from build123d import *

# Parameters (mm, degrees)
SKETCH1_R           = 11
BOSS_EXTRUDE2_DEPTH = 7


with BuildPart() as part:
    # Sketch1 → Boss-Extrude2 (new body)
    with BuildSketch(Plane.XY):
        with BuildLine():
            ThreePointArc((20.169463689, 41.588983826), (18.10306117, 49.087649082), (10.604395914, 47.021246564))
            Line((10.604395914, 47.021246564), (-12.118876528, 7.010361333))
            ThreePointArc((-12.118876528, 7.010361333), (-19.668266357, -0.440838827), (-29.907048562, -3.212302261))
            Line((-29.907048562, -3.212302261), (-46.101848355, -3.327223978))
            ThreePointArc((-46.101848355, -3.327223978), (-51.562681703, -8.866113681), (-46.023791999, -14.326947029))
            Line((-46.023791999, -14.326947029), (-0.01171274, -14.000435605))
            ThreePointArc((-0.01171274, -14.000435605), (10.215910802, -16.8127989), (17.735459644, -24.294112676))
            Line((17.735459644, -24.294112676), (25.932384666, -38.261759848))
            ThreePointArc((25.932384666, -38.261759848), (33.459620532, -40.221535401), (35.419396085, -32.694299535))
            Line((35.419396085, -32.694299535), (12.130589268, 6.990074273))
            ThreePointArc((12.130589268, 6.990074273), (9.452355555, 17.253637727), (12.171588918, 27.506414937))
            Line((12.171588918, 27.506414937), (20.169463689, 41.588983826))
        make_face()
        with BuildLine():
            Line((6.354309168, 34.829758236), (12.626103421, 45.873063758))
            ThreePointArc((12.626103421, 45.873063758), (16.954878364, 47.065941576), (18.147756182, 42.737166632))
            Line((18.147756182, 42.737166632), (11.875961929, 31.69386111))
            ThreePointArc((11.875961929, 31.69386111), (7.547186985, 30.500983292), (6.354309168, 34.829758236))
        make_face(mode=Mode.SUBTRACT)
        with BuildLine():
            ThreePointArc((-46.040290274, -12.002005566), (-49.23774024, -8.849615406), (-46.08535008, -5.652165441))
            Line((-46.08535008, -5.652165441), (-33.38566983, -5.56204583))
            ThreePointArc((-33.38566983, -5.56204583), (-30.188219864, -8.71443599), (-33.340610024, -11.911885955))
            Line((-33.340610024, -11.911885955), (-46.040290274, -12.002005566))
        make_face(mode=Mode.SUBTRACT)
        Circle(SKETCH1_R, mode=Mode.SUBTRACT)
        with BuildLine():
            ThreePointArc((33.414186854, -33.871058192), (32.282861875, -38.216326169), (27.937593898, -37.085001191))
            Line((27.937593898, -37.085001191), (21.509707901, -26.13181528))
            ThreePointArc((21.509707901, -26.13181528), (22.641032879, -21.786547303), (26.986300856, -22.917872281))
            Line((26.986300856, -22.917872281), (33.414186854, -33.871058192))
        make_face(mode=Mode.SUBTRACT)
    extrude(amount=BOSS_EXTRUDE2_DEPTH)


solid = part.part
Build history of the part. All positions in model axes, mm. A direction names the side the tool comes from. Round coordinates to 2 decimals unless told otherwise and drop trailing zeros. Order: outer loops, then holes, each group sorted by start corner. A loop starts at its lowest first (then second) coordinate and runs counter-clockwise, first axis right, second up. Notation, with made-up numbers: M 12.25,51.5 L 34.25,51.5 A29 cw 34.25,80.5 Z; hole C -37.5,-5 d1. An arc over 180 degrees is marked long. Use CSV: the item, a comma, the result in double quotes. Start each with the question number.
(1) Drill centre lines: probe 1 along Y at (x, z) = (-45, 1.5); probe 2 along Y at (x, z) = (0, 2.5); probe 3 along Y at (x, z) = (6.5, 3). Where is each one in solid material? Low to high.
(2) Mould opens along Y. For faces 4 (the face through (21.777, -31.18, 3.451)), 5 (the face through (-19.538, -0.366, 3.451)), 6 (the face through (9.446, 40.274, 3.451)), 7 (the face through (-51.562, -8.745, 3.451)) say: +Y half, -Y half, draft (parallel to the pull), parting line (faces both ways), or undercut.
(3) Tool access for faces 1 (the face through (-0.598, 27.296, 3.451)), 2 (the face through (23.94, -13.13, 3.45)), 3 (the face through (24.77, -31.69, 3.45)): list every direction of +Z, -Z, +X, -X, +Y, -Y with a clear straight run to the whole face (end or side of a thin tool).
(4) Flat gauge pins, fed straight in: P1, Ø10, axis at x = 17, y = 11, coming from the +Z side; P2, Ø1.5, axis at y = 36.5, z = 4, coming from the +X side; P3, Ø1, axis at y = 33, z = 1, coming from the -X side; P4, Ø2, axis at x = 8.5, z = 3.5, coming from the +Y side. Where does each tip first touch, or does it go through?
(5) Cut at D-D on x = -25.5. List the corners of the cut face in (y, z), then the cut area to 3 significant figures.
(6) Cut at B-B on y = 2. List the corners of the cut face in (x, z), then the cut area to 3 significant figures.
(7) Cut at C-C on x = 4. List the corners of the cut face in (y, z), then the cut area to 3 significant figures.
(8) Cut at A-A on z = 3.25. List the corners of the cut face in (x, y) (3 decimals).
Findings:
1,probe 1,"y = -14.32 to -11.99, -5.64 to -3.32"
1,probe 2,"y = -14 to -11, 11 to 28.35"
1,probe 3,"y = -15.12 to -8.87, 8.87 to 31.46, 35.09 to 39.79"
2,face 4,"-Y half"
2,face 5,"+Y half"
2,face 6,"undercut"
2,face 7,"parting line"
3,face 1,"+Z, -Z, -X, +Y"
3,face 2,"+Z, -Z, +X"
3,face 3,"+Z, -Z"
4,P1,"passes through"
4,P2,"stops at x = 17.71"
4,P3,"stops at x = 2.36"
4,P4,"stops at y = 45.08"
5,outline,"M -14.18,0 L -2.71,0 L -2.71,7 L -14.18,7 Z"
5,area,"80.3 mm^2"
6,outline,"M -16.27,0 L -10.82,0 L -10.82,7 L -16.27,7 Z; M 10.82,0 L 15.06,0 L 15.06,7 L 10.82,7 Z"
6,area,"67.8 mm^2"
7,outline,"M -14.44,0 L -10.25,0 L -10.25,7 L -14.44,7 Z; M 10.25,0 L 35.39,0 L 35.39,7 L 10.25,7 Z"
7,area,"205 mm^2"
8,outline,"M -46.102,-3.327 A5.5 ccw -46.024,-14.327 L -0.012,-14 A20.846 cw 17.735,-24.294 L 25.932,-38.262 A5.5 ccw 35.419,-32.694 L 12.131,6.99 A20.846 cw 12.172,27.506 L 20.169,41.589 A5.5 ccw 10.604,47.021 L -12.119,7.01 A20.846 cw -29.907,-3.212 Z; hole M -46.085,-5.652 A3.175 ccw -46.04,-12.002 L -33.341,-11.912 A3.175 ccw -33.386,-5.562 Z; hole C 0,0 d22; hole M 6.354,34.83 A3.175 ccw 11.876,31.694 L 18.148,42.737 A3.175 ccw 12.626,45.873 Z; hole M 21.51,-26.132 L 27.938,-37.085 A3.175 ccw 33.414,-33.871 L 26.986,-22.918 A3.175 ccw Z"
